from build123d import *

# Parameters (mm, degrees)
F1_DEPTH = 2.54
F2_R     = 0.508


with BuildPart() as f1:
    # F0 (on Front) → F1 (new body)
    with BuildSketch(Plane.XZ):
        with BuildLine():
            ThreePointArc((22.872963, 1.371057), (9.798592, 8.238838), (1.282963, 20.304891))
            ThreePointArc((1.282963, 20.304891), (0.583696, 22.247186), (0.012963, 24.231057))
            ThreePointArc((0.012963, 24.231057), (-8.419151, 9.803172), (-22.847037, 1.371057))
            ThreePointArc((-22.847037, 1.371057), (-8.637784, -7.27969), (0.012963, -21.488943))
            ThreePointArc((0.012963, -21.488943), (8.403265, -7.019245), (22.872963, 1.371057))
        make_face()
        with BuildLine():
            ThreePointArc((1.282963, -10.839783), (0.333154, -14.200904), (0.012963, -17.678943))
            ThreePointArc((0.012963, -17.678943), (-0.307228, -14.200904), (-1.257037, -10.839783))
            ThreePointArc((-1.257037, -10.839783), (-8.252406, -1.975623), (-19.037037, 1.371057))
            ThreePointArc((-19.037037, 1.371057), (-8.252406, 4.717738), (-1.257037, 13.581898))
            ThreePointArc((-1.257037, 13.581898), (-0.307228, 16.943019), (0.012963, 20.421057))
            ThreePointArc((0.012963, 20.421057), (0.333154, 16.943019), (1.282963, 13.581898))
            ThreePointArc((1.282963, 13.581898), (8.278332, 4.717738), (19.062963, 1.371057))
            ThreePointArc((19.062963, 1.371057), (8.278332, -1.975623), (1.282963, -10.839783))
        make_face(mode=Mode.SUBTRACT)
    extrude(amount=F1_DEPTH)

    # F2
    f2_edges = [f1.edges().sort_by_distance(p)[0] for p in [
        (0.012963, -1.27, 24.231057),
        (22.872963, -1.27, 1.371057),
        (0.012963, -1.27, -21.488943),
        (-22.847037, -1.27, 1.371057),
    ]]
    fillet(f2_edges, radius=F2_R)


solid = f1.part
Verification items for the finished model (mm, model axes). Give positions to 0.01 mm unless a question says otherwise; leave off trailing zeros. Write each loop counter-clockwise with the first axis right and the second up, starting at its lowest first coordinate (ties: lowest second). Pieces come first, ordered by that corner, then holes. Notation, with made-up numbers: M -1,-17 L 43,-17 A11 cw 43,1 Z; hole C -13,39 d10. An arc over 180 degrees is marked long. Put each result on its own line as item: value. Start each with the question number.
1. Section check A-A (x = 7.5). Record the cut outline in (y, z), and give its area (3 significant figures).
2. Scan lines: line 1 along X through (y, z) = (-1.1, 5); line 2 along Z through (x, y) = (-13.5, -1.15); line 3 along Z through (x, y) = (5, -0.95). Record each from-to range of solid material in increasing order. Write a range as [from, to].
3. Section check B-B (z = 5.5). Record the cut outline in (x, y).
4. Draft check along X on faces 1 (the face through (-8.32, -1.25, 9.9)), 2 (the face through (-5, -2.54, 8)), 3 (the face through (9.301, -1.252, 8.685)). Enter one of: +X half, -X half, draft (parallel to the pull), parting line (faces both ways), or undercut.
Answer list:
1. outline: M -2.54,-7.96 L 0,-7.96 L 0,-2.54 L -2.54,-2.54 Z; M -2.54,5.28 L 0,5.28 L 0,10.47 L -2.54,10.47 Z
1. area: 26.9 mm2
2. line 1: [-14.52, -7.85], [7.88, 14.21]
2. line 2: [-3.22, 0.55], [2.19, 5.65]
2. line 3: [-11.02, -4.83], [7.57, 13.52]
3. outline: M -13.72,-2.54 L -7.19,-2.54 L -7.19,0 L -13.72,0 Z; M 7.22,-2.54 L 13.42,-2.54 L 13.42,0 L 7.22,0 Z
4. face 1: -X half
4. face 2: draft
4. face 3: +X half
